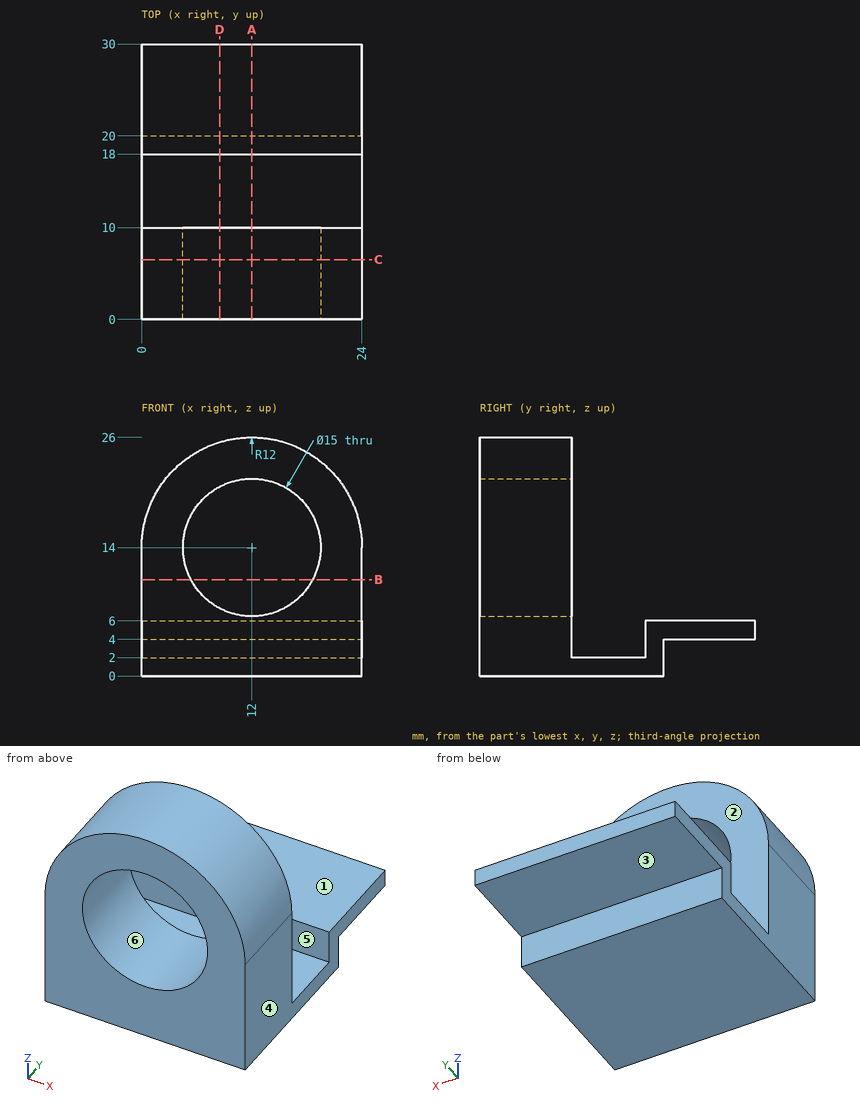
Source: three-view drawing plus pictorial views. Frame: mm from the lowest corner of the part. A direction names the side the tool comes from. Round coordinates to 2 decimals unless told otherwise and drop trailing zeros. Loops run counter-clockwise (first coordinate to the right, second up) from the corner with the lowest first, then second, coordinate; pieces in that order, holes last. Notation, with made-up numbers: M 61.25,18 L 88.25,18 A20 cw 88.25,48 Z; hole C 88,36.25 d10. An arc over 180 degrees is marked long. Put each result on its own line as item: value. Start each with the question number.
(1) Section query A-A (x = 12). Return loops of the section in (y, z), then the cut area to 3 significant figures.
(2) Set-up query: the marked faces 1, 2 and 3. Return all of +Z, -Z, +X, -X, +Y, -Y with unobstructed straight access to the full face (end or side cutting, diameter ignored); none if empty.
(3) Section query B-B (z = 10.5). Return loops of the section in (x, y).
(4) Section query D-D (x = 8.5). Return loops of the section in (y, z).
(5) Material intervals for line 1 along Z through (x, y) = (12, 7); line 2 along Y through (x, z) = (2.5, 5.5); line 3 along X through (y, z) = (7.5, 14), sorted ascending. Write a range as [from, to].
(6) Contact query for flat-ended pins moving along their axis: pin 1 Ø12 at (x, z) = (20, 16) entering from +Y; pin 2 Ø3 at (x, z) = (12.5, 2) entering from +Y; pin 3 Ø3 at (x, y) = (6.5, 22.5) entering from -Z. Output: stop coordinate, or through.
(7) Draft query along X for the marked faces 4, 5 and 6. Return one class per face: +X half, -X half, draft (parallel to the pull), parting line (faces both ways), or undercut.
(8) Section query C-C (y = 6.5). Return loops of the section in (x, z).
Findings below:
1. outline: M 0,0 L 20,0 L 20,4 L 30,4 L 30,6 L 18,6 L 18,2 L 10,2 L 10,6.5 L 0,6.5 Z; M 0,21.5 L 10,21.5 L 10,26 L 0,26 Z
1. area: 158 mm2
2. face 1: +Z, +X, -X, +Y
2. face 2: +Z, +X, -X
2. face 3: -Z, +X, -X, +Y
3. outline: M 0,0 L 5.37,0 L 5.37,10 L 0,10 Z; M 18.63,0 L 24,0 L 24,10 L 18.63,10 Z
4. outline: M 0,0 L 20,0 L 20,4 L 30,4 L 30,6 L 18,6 L 18,2 L 10,2 L 10,7.37 L 0,7.37 Z; M 0,20.63 L 10,20.63 L 10,25.48 L 0,25.48 Z
5. line 1: z = [0, 6.5], [21.5, 26]
5. line 2: y = [0, 10], [18, 30]
5. line 3: x = [0, 4.5], [19.5, 24]
6. pin 1: stops at y = 10
6. pin 2: stops at y = 20
6. pin 3: stops at z = 4
7. face 4: +X half
7. face 5: draft
7. face 6: undercut
8. outline: M 0,0 L 24,0 L 24,14 A12 ccw 0,14 Z; hole C 12,14 d15
